from build123d import *

# Parameters (mm, degrees)
FILLET1_R = 1


with BuildPart() as part:
    # Sketch1 → Revolve1 (revolve)
    with BuildSketch(Plane.XY):
        Polygon((-4, -20), (-4, 0), (-11, 0), (-11, 1.5), (-10, 1.5), (-10, 11), (-11, 11), (-11, 12.5), (0, 12.5), (0, -20), align=None)
    revolve(axis=Axis((0, 12.5, 0), (0, -1, 0)))

    # Fillet1
    fillet1_edges = [part.edges().sort_by_distance(p)[0] for p in [
        (4, -20, 0),
    ]]
    fillet(fillet1_edges, radius=FILLET1_R)


solid = part.part
Check sheet for the modelled part. Datum: model origin and axes. Units: mm. A direction names the side the tool comes from. Round coordinates to 2 decimals unless told otherwise and drop trailing zeros. Loops run counter-clockwise (first coordinate to the right, second up) from the corner with the lowest first, then second, coordinate; pieces in that order, holes last. Notation, with made-up numbers: M 87,37.5 L 114,37.5 A26 ccw 114,59.5 Z; hole C 67.5,-23 d2. An arc over 180 degrees is marked long. One line per question, with ' | ' between items. Start each with the question number.
Item 1: Set-up check for faces 1 (the face through (-2, 1.5, 10)), 2 (the face through (0, 12.5, 0)), 3 (the face through (0.867, -9.367, 3.905)): record each of +Z, -Z, +X, -X, +Y, -Y from which the full face is reachable in a straight line by a thin tool's end or side.
Item 2: Section check B-B (x = 0). Record the boundary of the cut face in (y, z), and give its area (3 significant figures).
Item 3: Scan lines: probe 1 along Y at (x, z) = (-8.5, 6); probe 2 along Y at (x, z) = (1, -5); probe 3 along X at (y, z) = (-4.5, -0.25). Record each from-to range of solid material in increasing order.
Item 4: Section check C-C (y = -13). Record the boundary of the cut face in (x, z), and give its area (3 significant figures).
Item 5: Section check D-D (x = 5). Record the boundary of the cut face in (y, z), and give its area (3 significant figures).
Item 6: Section check A-A (z = 0). Record the boundary of the cut face in (x, y).
Item 7: Gauge pin test, flat ends, axial feed: pin 1 Ø5 at (x, z) = (1.5, -6.5) entering from -Y; pin 2 Ø2 at (y, z) = (1, 3.5) entering from -X; pin 3 Ø6.5 at (x, z) = (3, -4.5) entering from -Y; pin 4 Ø6 at (x, y) = (4.5, 9) entering from +Z. Record the tip position at first contact, or that the pin passes through.
Worked out:
1) face 1: none | face 2: +Z, -Z, +X, -X, +Y | face 3: -Y
2) outline: M -20,-3 A1 ccw -19,-4 L 0,-4 L 0,-11 L 1.5,-11 L 1.5,-10 L 11,-10 L 11,-11 L 12.5,-11 L 12.5,11 L 11,11 L 11,10 L 1.5,10 L 1.5,11 L 0,11 L 0,4 L -19,4 A1 ccw -20,3 Z | area: 416 mm^2
3) probe 1: 0 to 1.5, 11 to 12.5 | probe 2: 0 to 12.5 | probe 3: -3.99 to 3.99
4) outline: C 0,0 d8 | area: 50.3 mm^2
5) outline: M 0,-9.8 L 1.5,-9.8 L 1.5,-8.66 L 11,-8.66 L 11,-9.8 L 12.5,-9.8 L 12.5,9.8 L 11,9.8 L 11,8.66 L 1.5,8.66 L 1.5,9.8 L 0,9.8 Z | area: 223 mm^2
6) outline: M -11,0 L -4,0 L -4,-19 A1 ccw -3,-20 L 3,-20 A1 ccw 4,-19 L 4,0 L 11,0 L 11,1.5 L 10,1.5 L 10,11 L 11,11 L 11,12.5 L -11,12.5 L -11,11 L -10,11 L -10,1.5 L -11,1.5 Z
7) pin 1: y = 0 | pin 2: x = -10.71 | pin 3: y = -20 | pin 4: z = 10.76
